```python
from build123d import *

# Parameters (mm, degrees)
F0_W     = 1
F0_H     = 15
F1_DEPTH = 20


with BuildPart() as f1:
    # F0 (on Top) → F1 (new body)
    with BuildSketch(Plane.XY):
        Polygon((31.285321, 24.755745), (-2.714679, 24.755745), (-14.714679, 14.755745), (-14.714679, -5.244255), (-4.714679, -5.244255), (-3.714679, -5.244255), (31.285321, -5.244255), align=None)
        with Locations((-4.214679, -12.744255)):
            Rectangle(F0_W, F0_H)
    extrude(amount=F1_DEPTH)


solid = f1.part
```
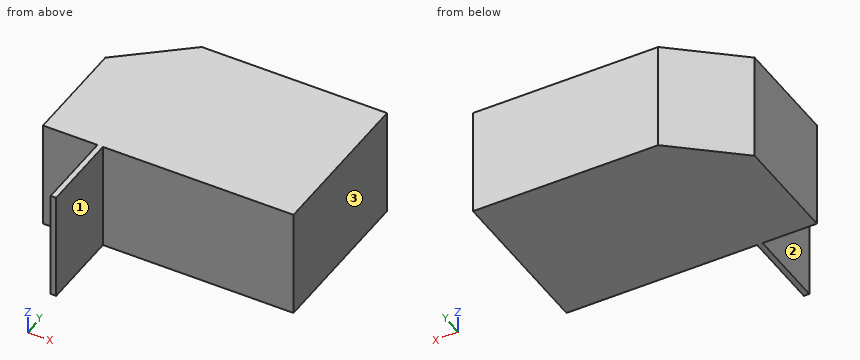
Could you check a few things on this model? Use its own coordinates, in mm. Face numbers are marked on the shaded views. A direction names the side the tool comes from. Round coordinates to 2 decimals unless told otherwise and drop trailing zeros. Loops run counter-clockwise (first coordinate to the right, second up) from the corner with the lowest first, then second, coordinate; pieces in that order, holes last. Notation, with made-up numbers: M 14.5,23 L 56.5,23 A26 ccw 56.5,43 Z; hole C 66.5,63 d2. An arc over 180 degrees is marked long. Write item = value, one per line.
1. I want a section at C-C, the plane x = 21.5. Write out the boundary of the cut face in (y, z), and give its area (3 significant figures).
Results below:
outline = M -5.24,0 L 24.76,0 L 24.76,20 L -5.24,20 Z
area = 600 mm²
2. Which directions (+Z, -Z, +X, -X, +Y, -Y) give clear straight access to the entire face, cutting with the end or side of a thin tool? Please do the marked faces 1, 2 and 3.
Results below:
face_1 = +Z, -Z, +X, -Y
face_2 = +Z, -Z, -X, -Y
face_3 = +Z, -Z, +X, +Y, -Y
3. I want a section at A-A, the plane z = 8.5. Write out the boundary of the cut face in (x, y), and give its area (4 significant figures).
Results below:
outline = M -14.71,-5.24 L -4.71,-5.24 L -4.71,-20.24 L -3.71,-20.24 L -3.71,-5.24 L 31.29,-5.24 L 31.29,24.76 L -2.71,24.76 L -14.71,14.76 Z
area = 1,335 mm²
4. I need wall thicknesses on probe 1 along Y at (x, z) = (-1, 1.5); probe 2 along X at (y, z) = (-6, 12.5); probe 3 along Y at (x, z) = (-8, 15.25). Which ranges of each line are inside material? Lowest first, please.
Results below:
probe_1 = -5.24 to 24.76
probe_2 = -4.71 to -3.71
probe_3 = -5.24 to 20.35
5. I want a section at B-B, the plane y = -16. Write out the boundary of the cut face in (x, z).
Results below:
outline = M -4.71,0 L -3.71,0 L -3.71,20 L -4.71,20 Z
6. Will these pins go through, and if not, where does the flat tip stop? P1, Ø4.5, axis at y = -11.5, z = 8, coming from the +X side; P2, Ø5, axis at x = -6, z = 7.5, coming from the +Y side; P3, Ø3, axis at x = -10.5, z = 10.5, coming from the -Y side.
Results below:
P1 = -3.71
P2 = 24.1
P3 = -5.24
